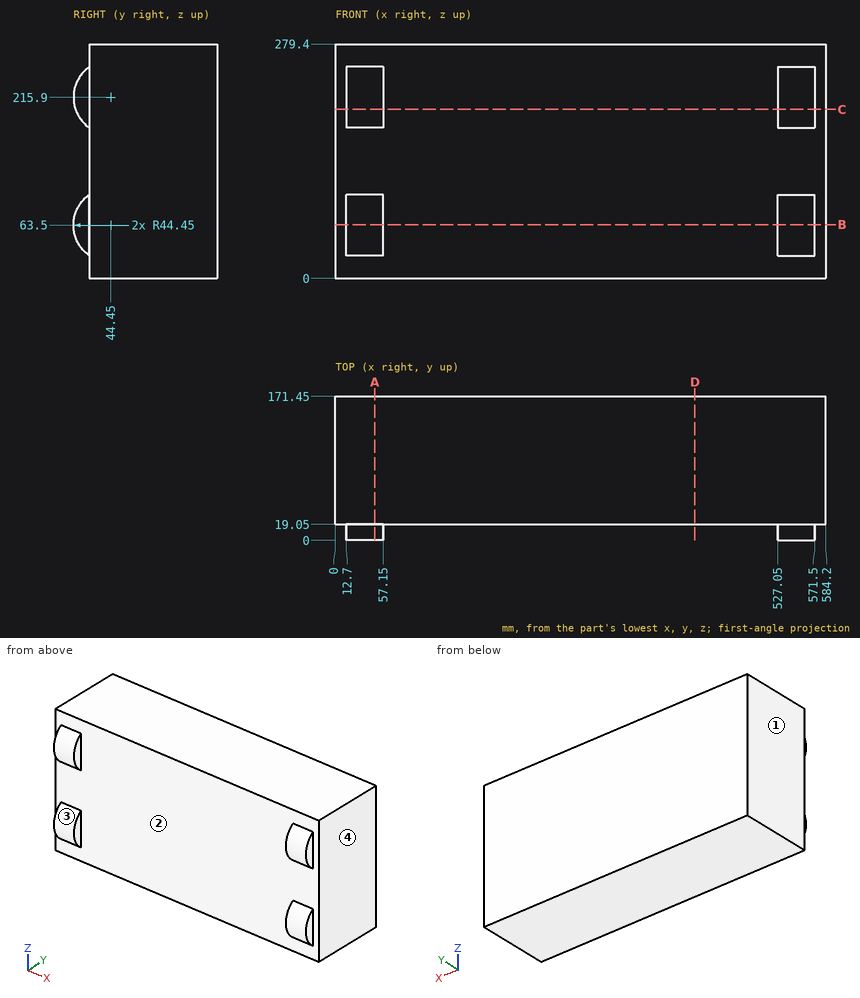
Input: dimensioned drawing with shaded views. Units: mm. Origin: part minimum x, y, z. Coordinates: 2 decimals unless noted, no trailing zeros. Write each loop counter-clockwise with the first axis right and the second up, starting at its lowest first coordinate (ties: lowest second). Pieces come first, ordered by that corner, then holes. Notation, with made-up numbers: M -27.5,73 L -7.5,73 A10 cw -7.5,92 Z; hole C 80,-9 d1. An arc over 180 degrees is marked long. Answer as a JSON object with one key per item and string values. Group by question number.
(1) Ray query, line 1 along Y through (x, z) = (422, 157); line 2 along Y through (x, z) = (36.5, 64). Return the intervals inside material, ascending. Write a range as [from, to].
(2) Section B-B on z = 64. Output: boundary loops of the cut face in (x, y), plus the area to 3 significant figures.
(3) Contact query for flat-ended pins moving along their axis: P1, Ø9.5, axis at y = 12.5, z = 77.5, coming from the -X side; P2, Ø21, axis at y = 5.5, z = 204, coming from the +X side; P3, Ø2, axis at x = 425, z = 218.5, coming from the -Y side. Output: stop coordinate, or through.
(4) Section C-C on z = 201.5. Output: boundary loops of the cut face in (x, y), plus the area to 3 significant figures.
(5) Section A-A on x = 47. Output: boundary loops of the cut face in (y, z).
(6) Section D-D on x = 428.5. Output: boundary loops of the cut face in (y, z), plus the area to 3 significant figures.
(7) Mould query, pull axis X, two halves, no side actions, for the marked faces 1, 2, 3 and 4. Classes: pulls with the +X half, pulls with the -X half, needs draft (parallel to the pull), parting line crosses it, or undercut.
Result set:
{
 "1": {"line 1": "y = [19.05, 171.45]", "line 2": "y = [0, 171.45]"},
 "2": {"outline": "M 0,19.05 L 12.7,19.05 L 12.7,0 L 57.15,0 L 57.15,19.05 L 527.05,19.05 L 527.05,0 L 571.5,0 L 571.5,19.05 L 584.2,19.05 L 584.2,171.45 L 0,171.45 Z", "area": "90,700 mm2"},
 "3": {"P1": "stops at x = 12.7", "P2": "stops at x = 571.5", "P3": "stops at y = 19.05"},
 "4": {"outline": "M 0,19.05 L 12.7,19.05 L 12.7,2.4 L 57.15,2.4 L 57.15,19.05 L 527.05,19.05 L 527.05,2.4 L 571.5,2.4 L 571.5,19.05 L 584.2,19.05 L 584.2,171.45 L 0,171.45 Z", "area": "90,500 mm2"},
 "5": {"outline": "M 19.05,0 L 171.45,0 L 171.45,279.4 L 19.05,279.4 L 19.05,252.38 A44.45 ccw 19.05,179.42 L 19.05,99.98 A44.45 ccw 19.05,27.02 Z"},
 "6": {"outline": "M 19.05,0 L 171.45,0 L 171.45,279.4 L 19.05,279.4 Z", "area": "42,600 mm2"},
 "7": {"face 1": "pulls with the -X half", "face 2": "undercut", "face 3": "needs draft", "face 4": "pulls with the +X half"}
}
